Could you check a few things on this model? Use its own coordinates, in mm. Face numbers are marked on the shaded views. A direction names the side the tool comes from. Coordinates: 2 decimals unless noted, no trailing zeros. Write each loop counter-clockwise with the first axis right and the second up, starting at its lowest first coordinate (ties: lowest second). Pieces come first, ordered by that corner, then holes. Notation, with made-up numbers: (-24, 41.25) - (1, 41.25) arc R21 cw to (1, 72.25) - close; hole circle Ø10 at (-13, 17). An arc over 180 degrees is marked (long way). Write item = value, one per line. Start each with the question number.
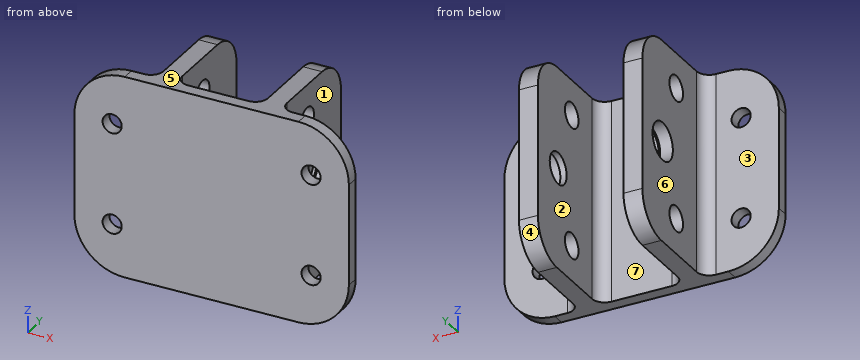
```python
from build123d import *

# Parameters (mm, degrees)
BOSS_EXTRUDE2_DEPTH = 50.8
SKETCH4_R           = 3.175
SKETCH4_R_2         = 3.96875
CUT_EXTRUDE1_DEPTH  = 51.165
SKETCH5_R           = 2.413
CUT_EXTRUDE2_DEPTH  = 4.175
SKETCH4_3_R         = 4.7625
SKETCH4_3_R_2       = 3.96875
CUT_EXTRUDE3_DEPTH  = 3.175
SKETCH6_R           = 4.7625
SKETCH6_R_2         = 3.96875
CUT_EXTRUDE4_DEPTH  = 3.175
FILLET1_R           = 12.7
FILLET2_R           = 3.175
FILLET3_R           = 8.89


with BuildPart() as part:
    # Sketch3 → Boss-Extrude2 (new body)
    with BuildSketch(Plane.XY):
        Polygon((-34.6075, 0), (34.6075, 0), (34.6075, 3.175), (15.5575, 3.175), (15.5575, 31.75), (10.795, 31.75), (10.795, 3.175), (-10.795, 3.175), (-10.795, 31.75), (-15.5575, 31.75), (-15.5575, 3.175), (-34.6075, 3.175), align=None)
    extrude(amount=BOSS_EXTRUDE2_DEPTH)

    # Sketch4 → Cut-Extrude1 (cut, through all)
    with BuildSketch(Plane.ZY.offset(15.5575)):
        with Locations((8.89, 15.875)):
            Circle(SKETCH4_R)
        with Locations((41.91, 15.875)):
            Circle(SKETCH4_R)
        with Locations((25.4, 22.225)):
            Circle(SKETCH4_R_2)
    extrude(amount=-CUT_EXTRUDE1_DEPTH, mode=Mode.SUBTRACT)

    # Sketch5 → Cut-Extrude2 (cut, through all)
    with BuildSketch(Plane(origin=(0, 3.175, 0), x_dir=(1, 0, 0), z_dir=(0, 1, 0))):
        with Locations((-25.0825, -38.1)):
            Circle(SKETCH5_R)
        with Locations((-25.0825, -12.7)):
            Circle(SKETCH5_R)
        with Locations((25.0825, -12.7)):
            Circle(SKETCH5_R)
        with Locations((25.0825, -38.1)):
            Circle(SKETCH5_R)
    extrude(amount=-CUT_EXTRUDE2_DEPTH, mode=Mode.SUBTRACT)

    # Sketch4_3 → Cut-Extrude3 (cut)
    with BuildSketch(Plane.ZY.offset(15.5575)):
        with Locations((25.4, 22.225)):
            Circle(SKETCH4_3_R)
        with Locations((25.4, 22.225)):
            Circle(SKETCH4_3_R_2, mode=Mode.SUBTRACT)
    extrude(amount=-CUT_EXTRUDE3_DEPTH, mode=Mode.SUBTRACT)

    # Sketch6 → Cut-Extrude4 (cut)
    with BuildSketch(Plane(origin=(15.5575, 0, 0), x_dir=(0, 0, -1), z_dir=(1, 0, 0))):
        with Locations((-25.4, 22.225)):
            Circle(SKETCH6_R)
        with Locations((-25.4, 22.225)):
            Circle(SKETCH6_R_2, mode=Mode.SUBTRACT)
    extrude(amount=-CUT_EXTRUDE4_DEPTH, mode=Mode.SUBTRACT)

    # Fillet1
    fillet1_edges = [part.edges().sort_by_distance(p)[0] for p in [
        (34.6075, 1.5875, 50.8),
        (34.6075, 1.5875, 0),
        (-34.6075, 1.5875, 0),
        (-34.6075, 1.5875, 50.8),
    ]]
    fillet(fillet1_edges, radius=FILLET1_R)

    # Fillet2
    fillet2_edges = [part.edges().sort_by_distance(p)[0] for p in [
        (-15.5575, 3.175, 25.4),
        (-10.795, 3.175, 25.4),
        (10.795, 3.175, 25.4),
        (15.5575, 3.175, 25.4),
    ]]
    fillet(fillet2_edges, radius=FILLET2_R)

    # Fillet3
    fillet3_edges = [part.edges().sort_by_distance(p)[0] for p in [
        (-13.17625, 31.75, 0),
        (13.17625, 31.75, 0),
        (13.17625, 31.75, 50.8),
        (-13.17625, 31.75, 50.8),
    ]]
    fillet(fillet3_edges, radius=FILLET3_R)


solid = part.part
```
1) If I drill on probe 1 along X at (y, z) = (1, 38); probe 2 along X at (y, z) = (22.5, 16) (1 decimal); probe 3 along Y at (x, z) = (-14, 25), over which ranges is the centre line in solid material (lowest first)? Write a range as [from, to].
2) Suppose I cut it at C-C on x = -26. Please give me the cut outline in (y, z) (3 decimals), plus the area to 3 significant figures.
3) Which directions (+Z, -Z, +X, -X, +Y, -Y) give clear straight access to the entire face, cutting with the end or side of a thin tool? Please do the marked faces 1, 2, 3 and 4.
4) For P1, Ø12, axis at y = 14.5, z = 8.5, coming from the +X side; P2, Ø10, axis at y = 15.875, z = 41.91, coming from the -X side; P3, Ø4.5, axis at x = 1, z = 26.5, coming from the +Y side (3 decimals), each with a flat end and sliding along its axis, tell me the tip position at first contact or that it passes through.
5) Thinking about a two-plate mould opening in X: for the marked faces 5, 6 and 7, which applies, +X half, -X half, draft (parallel to the pull), parting line (faces both ways), or undercut?
6) Suppose I cut it at B-B on z = 25.4. State how many separate pieces and enclosed holes the cut face has, plus the area to 3 significant figures.
7) Suppose I cut it at A-A on y = 9. Please give me the cut outline in (x, z) (1 decimal), plus the area to 3 significant figures.
Reply:
q1.probe_1 = [-34.61, -27.49], [-22.67, 22.67], [27.49, 34.61]
q1.probe_2 = [-15.6, -10.8], [10.8, 15.6]
q1.probe_3 = [0, 17.48], [26.97, 31.75]
q2.outline = (0, 0.677) - (3.175, 0.677) - (3.175, 10.468) - (0, 10.468) - close; (0, 14.932) - (3.175, 14.932) - (3.175, 35.868) - (0, 35.868) - close; (0, 40.332) - (3.175, 40.332) - (3.175, 50.123) - (0, 50.123) - close
q2.area = 129 mm^2
q3.face_1 = +Z, -Z, +X, +Y
q3.face_2 = +Z, -Z, +Y
q3.face_3 = +Z, -Z, -X, +Y
q3.face_4 = -Z, +X, -X, +Y
q4.P1 = 15.56
q4.P2 = -15.56
q4.P3 = 3.175
q5.face_5 = draft
q5.face_6 = -X half
q5.face_7 = undercut
q6.separate_pieces = 3
q6.enclosed_holes = 0
q6.area = 415 mm^2
q7.outline = (-15.6, 0) - (-10.8, 0) - (-10.8, 50.8) - (-15.6, 50.8) - close; (10.8, 0) - (15.6, 0) - (15.6, 50.8) - (10.8, 50.8) - close
q7.area = 484 mm^2
